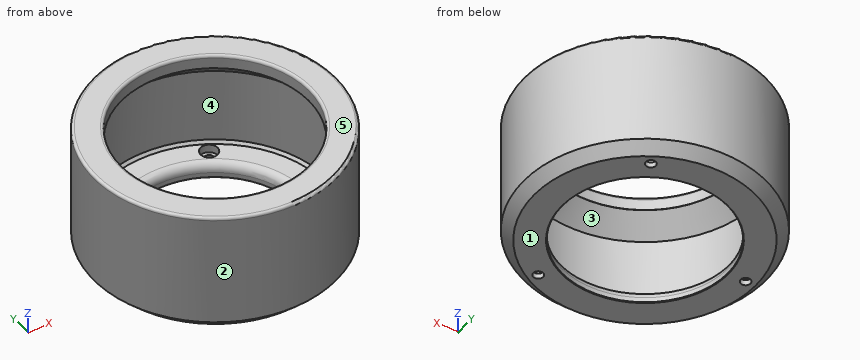
from build123d import *

# Parameters (mm, degrees)
SKETCH_R         = 44
SKETCH_R_2       = 30
PAD_DEPTH        = 5
SKETCH001_R      = 44
SKETCH001_R_2    = 41
PAD001_DEPTH     = 35
SKETCH002_R      = 44
SKETCH002_R_2    = 34
PAD002_DEPTH     = 5
HOLE_D           = 3.6
HOLE_DEPTH       = 5
HOLE_CBORE_D     = 6.2
HOLE_CBORE_DEPTH = 3
CHAMFER_SIZE     = 6.9
FILLET_R         = 1
CHAMFER001_SIZE  = 1
CHAMFER002_SIZE  = 3.8
FILLET001_R      = 3
CHAMFER003_SIZE  = 0.2


with BuildPart() as part:
    # Sketch → Pad (new body)
    with BuildSketch(Plane.XY):
        Circle(SKETCH_R)
        Circle(SKETCH_R_2, mode=Mode.SUBTRACT)
    extrude(amount=PAD_DEPTH)

    # Sketch001 (on DatumPlane) → Pad001 (join)
    with BuildSketch(Plane.XY.offset(5)):
        Circle(SKETCH001_R)
        Circle(SKETCH001_R_2, mode=Mode.SUBTRACT)
    extrude(amount=PAD001_DEPTH)

    # Sketch002 (on DatumPlane) → Pad002 (join)
    with BuildSketch(Plane.XY.offset(40)):
        Circle(SKETCH002_R)
        Circle(SKETCH002_R_2, mode=Mode.SUBTRACT)
    extrude(amount=PAD002_DEPTH)

    # Hole
    with Locations(Plane.XY.offset(5)):
        with Locations((-36.6, 0), (18.3, 31.69653), (18.3, -31.69653)):
            CounterBoreHole(HOLE_D / 2, HOLE_CBORE_D / 2, HOLE_CBORE_DEPTH, depth=HOLE_DEPTH)

    # Chamfer
    chamfer_edges = [part.edges().sort_by_distance(p)[0] for p in [
        (-41, 0, 40),
    ]]
    chamfer(chamfer_edges, length=CHAMFER_SIZE)

    # Fillet
    fillet_edges = [part.edges().sort_by_distance(p)[0] for p in [
        (-34, 0, 45),
        (-44, 0, 45),
    ]]
    fillet(fillet_edges, radius=FILLET_R)

    # Chamfer001
    chamfer001_edges = [part.edges().sort_by_distance(p)[0] for p in [
        (-41, 0, 5),
    ]]
    chamfer(chamfer001_edges, length=CHAMFER001_SIZE)

    # Chamfer002
    chamfer002_edges = [part.edges().sort_by_distance(p)[0] for p in [
        (-44, 0, 0),
    ]]
    chamfer(chamfer002_edges, length=CHAMFER002_SIZE)

    # Fillet001
    fillet001_edges = [part.edges().sort_by_distance(p)[0] for p in [
        (-30, 0, 5),
    ]]
    fillet(fillet001_edges, radius=FILLET001_R)

    # Chamfer003
    chamfer003_edges = [part.edges().sort_by_distance(p)[0] for p in [
        (-30, 0, 0),
    ]]
    chamfer(chamfer003_edges, length=CHAMFER003_SIZE)


solid = part.part
Can you work these out from the model? Positions are in its coordinate system, mm. Face numbers are marked on the shaded views. A direction names the side the tool comes from. Coordinates: 2 decimals unless noted, no trailing zeros. Loops run counter-clockwise (first coordinate to the right, second up) from the corner with the lowest first, then second, coordinate; pieces in that order, holes last. Notation, with made-up numbers: M -26.75,41.5 L -11.75,41.5 A26 cw -11.75,73.5 Z; hole C 71,17.5 d4. An arc over 180 degrees is marked long. Answer as CSV lines item,"result". Start each with the question number.
1. If I drill on probe 1 along Y at (x, z) = (18, 1); probe 2 along X at (y, z) = (14, 12); probe 3 along X at (y, z) = (30, 9), over which ranges is the centre line in solid material (lowest first)? Write a range as [from, to].
2. For the marked faces 4 and 5, which set-ups out of +Z, -Z, +X, -X, +Y, -Y let a thin tool reach every point of the face, with its end or its side?
3. Thinking about a two-plate mould opening in X: for the marked faces 1, 2 and 3, which applies, +X half, -X half, draft (parallel to the pull), parting line (faces both ways), or undercut?
4. Suppose I cut it at A-A, the plane y = 0. Count the separate pieces of the cut face and the enclosed holes in it, plus the area to 3 significant figures.
5. For pin 1 Ø1 at (y, z) = (15, 17.5) entering from +X; pin 2 Ø2 at (y, z) = (10, 40) entering from -X; pin 3 Ø8 at (y, z) = (17.5, 15.5) entering from +X, each with a flat end and sliding along its axis, tell me the tip position at first contact or that it passes through.
6. Suppose I cut it at B-B, the plane z = 27. List the corners of the cut face in (x, y) for me, plus the area to 3 significant figures.
Output:
1,probe 1,"y = [-37.06, -33.47], [-29.92, -24], [24, 29.92], [33.47, 37.06]"
1,probe 2,"x = [-41.71, -38.54], [38.54, 41.71]"
1,probe 3,"x = [-32.19, -27.95], [27.95, 32.19]"
2,face 4,"none"
2,face 5,"+Z, +X, -X, +Y, -Y"
3,face 1,"draft"
3,face 2,"parting line"
3,face 3,"undercut"
4,separate pieces,"3"
4,enclosed holes,"0"
4,area,"454 mm^2"
5,pin 1,"stops at x = 41.54"
5,pin 2,"stops at x = -43.07"
5,pin 3,"stops at x = 41.88"
6,outline,"C 0,0 d88; hole C 0,0 d82"
6,area,"801 mm^2"
